Could you check a few things on this model? Use its own coordinates, in mm. A direction names the side the tool comes from. Give positions to 0.01 mm unless a question says otherwise; leave off trailing zeros. Loops run counter-clockwise (first coordinate to the right, second up) from the corner with the lowest first, then second, coordinate; pieces in that order, holes last. Notation, with made-up numbers: M 83,-3.75 L 138,-3.75 A22 ccw 138,15.25 Z; hole C 26.25,17.5 d3. An arc over 180 degrees is marked long. Use CSV: the item, a comma, the result in double quotes.
```python
from build123d import *

# Parameters (mm, degrees)
SKETCH1_R           = 22.5
SKETCH1_R_2         = 1.6
SKETCH1_R_3         = 12.5
BOSS_EXTRUDE1_DEPTH = 4
SKETCH2_R           = 3
CUT_EXTRUDE1_DEPTH  = 2


with BuildPart() as part:
    # Sketch1 → Boss-Extrude1 (new body)
    with BuildSketch(Plane(origin=(0, 0, 0), x_dir=(1, 0, 0), z_dir=(0, 1, 0))):
        with Locations(Location((0, 0, 0), (0, 0, 270))):
            Circle(SKETCH1_R)
        with Locations(Location((0, 18, 0), (0, 0, 270))):
            Circle(SKETCH1_R_2, mode=Mode.SUBTRACT)
        with Locations(Location((15.588457268, 9, 0), (0, 0, 270))):
            Circle(SKETCH1_R_2, mode=Mode.SUBTRACT)
        with Locations(Location((15.588457268, -9, 0), (0, 0, 270))):
            Circle(SKETCH1_R_2, mode=Mode.SUBTRACT)
        with Locations(Location((0, -18, 0), (0, 0, 270))):
            Circle(SKETCH1_R_2, mode=Mode.SUBTRACT)
        with Locations(Location((-15.588457268, -9, 0), (0, 0, 270))):
            Circle(SKETCH1_R_2, mode=Mode.SUBTRACT)
        with Locations(Location((-15.588457268, 9, 0), (0, 0, 270))):
            Circle(SKETCH1_R_2, mode=Mode.SUBTRACT)
        with Locations(Location((0, 0, 0), (0, 0, 270))):
            Circle(SKETCH1_R_3, mode=Mode.SUBTRACT)
    extrude(amount=BOSS_EXTRUDE1_DEPTH)

    # Sketch2 → Cut-Extrude1 (cut)
    with BuildSketch(Plane(origin=(0, 4, 0), x_dir=(1, 0, 0), z_dir=(0, 1, 0))):
        with Locations(Location((-15.588457268, 9, 0), (0, 0, 270))):
            Circle(SKETCH2_R)
        with Locations(Location((15.588457268, 9, 0), (0, 0, 270))):
            Circle(SKETCH2_R)
        with Locations(Location((0, -18, 0), (0, 0, 270))):
            Circle(SKETCH2_R)
    extrude(amount=-CUT_EXTRUDE1_DEPTH, mode=Mode.SUBTRACT)


solid = part.part
```
1. If we mould it in two halves opening along Z, with no side actions, what happens to faces 3 (the face through (-8.618, 1.972, 20.784)), 4 (the face through (-10, 4, 10)), 5 (the face through (1.08, 0.99, 16.82)), 6 (the face through (-12.614, 3.014, -9.391))? For each: +Z half, -Z half, draft (parallel to the pull), parting line (faces both ways), or undercut.
Outcome:
face 3,"parting line"
face 4,"draft"
face 5,"undercut"
face 6,"undercut"
2. I want a section at A-A, the plane z = 18. List the corners of the cut face in (x, y) for me, then the cut area to 3 significant figures.
Outcome:
outline,"M -13.5,0 L -1.6,0 L -1.6,2 L -3,2 L -3,4 L -13.5,4 Z; M 1.6,0 L 13.5,0 L 13.5,4 L 3,4 L 3,2 L 1.6,2 Z"
area,"89.6 mm2"
3. I want a section at C-C, the plane y = 1.2. List the corners of the cut face in (x, z) for me.
Outcome:
outline,"C 0,0 d45; hole C -15.59,-9 d3.2; hole C -15.59,9 d3.2; hole C 0,0 d25; hole C 0,-18 d3.2; hole C 0,18 d3.2; hole C 15.59,-9 d3.2; hole C 15.59,9 d3.2"
4. I want a section at B-B, the plane x = 0. List the corners of the cut face in (y, z) for me, then the cut area to 3 significant figures.
Outcome:
outline,"M 0,-22.5 L 4,-22.5 L 4,-19.6 L 0,-19.6 Z; M 0,-16.4 L 4,-16.4 L 4,-12.5 L 0,-12.5 Z; M 0,12.5 L 4,12.5 L 4,15 L 2,15 L 2,16.4 L 0,16.4 Z; M 0,19.6 L 2,19.6 L 2,21 L 4,21 L 4,22.5 L 0,22.5 Z"
area,"48.8 mm2"
5. I'm going to push flat-ended pins straight in: pin 1 Ø1.9 at (x, z) = (0, -18) entering from -Y; pin 2 Ø3.5 at (x, z) = (15.59, -9) entering from +Y; pin 3 Ø1.5 at (y, z) = (3, 10) entering from +X; pin 4 Ø1 at (y, z) = (0.5, -7.5) entering from +X. Where does each tip first touch, or does it pass through?
Outcome:
pin 1,"through"
pin 2,"y = 2"
pin 3,"x = 20.51"
pin 4,"x = 21.38"
6. Please list where these lines run through material, in increasing order: line 1 (X direction, y = 1.75, z = 0); line 2 (X direction, y = 1.25, z = -10); line 3 (X direction, y = 1, z = -9).
Outcome:
line 1,"-22.5 to -12.5, 12.5 to 22.5"
line 2,"-20.16 to -16.84, -14.34 to -7.5, 7.5 to 14.34, 16.84 to 20.16"
line 3,"-20.62 to -17.19, -13.99 to -8.67, 8.67 to 13.99, 17.19 to 20.62"
7. I want a section at D-D, the plane x = 14.5. List the corners of the cut face in (y, z) for me.
Outcome:
outline,"M 0,-17.2 L 4,-17.2 L 4,-11.8 L 2,-11.8 L 2,-10.17 L 0,-10.17 Z; M 0,-7.83 L 2,-7.83 L 2,-6.2 L 4,-6.2 L 4,7.83 L 0,7.83 Z; M 0,10.17 L 4,10.17 L 4,17.2 L 0,17.2 Z"
8. Which directions (+Z, -Z, +X, -X, +Y, -Y) give clear straight access to the entire face, cutting with the end or side of a thin tool? Please do faces 1 (the face through (14.027, 0.986, -9.347)), 2 (the face through (-16.9, 2, -7.7)).
Outcome:
face 1,"+Y, -Y"
face 2,"+Y"
